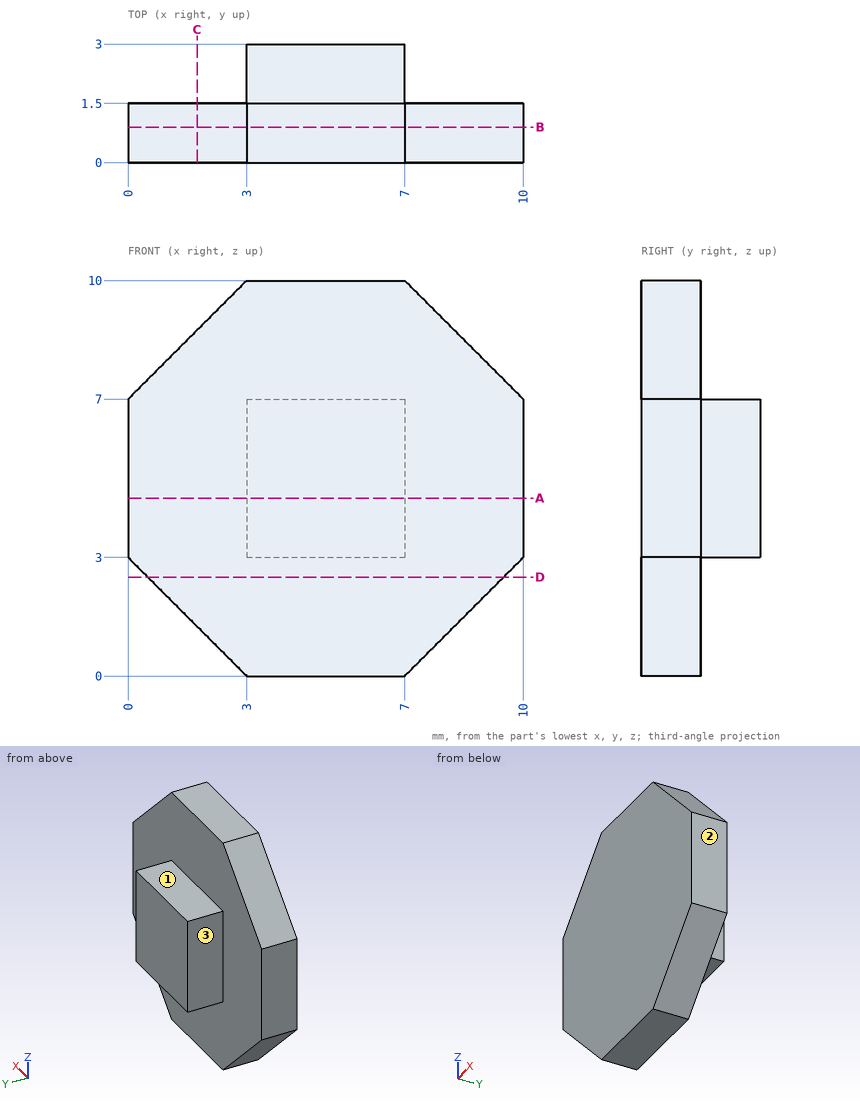
Could you check a few things on this drawing? It's one solid part, dimensions in mm from its lowest x, y, z. A direction names the side the tool comes from. Give positions to 0.01 mm unless a question says otherwise; leave off trailing zeros. Order: outer loops, then holes, each group sorted by start corner. A loop starts at its lowest first (then second) coordinate and runs counter-clockwise, first axis right, second up. Notation, with made-up numbers: M -31,54 L -6,54 A11 ccw -6,60 Z; hole C -31,-23 d7. An arc over 180 degrees is marked long. Use one line per item in the form item = value.
Item 1: If we section it at D-D, the plane z = 2.5: Write out the boundary of the cut face in (x, y), and give its area (3 significant figures).
Values follow:
outline = M 0.5,0 L 9.5,0 L 9.5,1.5 L 0.5,1.5 Z
area = 13.5 mm^2
Item 2: If I drill on line 1 along Y through (x, z) = (8.25, 1.75); line 2 along Z through (x, y) = (4.75, 2.45), over which ranges is the centre line in solid material (lowest first)? Write a range as [from, to].
Values follow:
line_1 = [0, 1.5]
line_2 = [3, 7]
Item 3: If we section it at C-C, the plane x = 1.75: Write out the boundary of the cut face in (y, z).
Values follow:
outline = M 0,1.25 L 1.5,1.25 L 1.5,8.75 L 0,8.75 Z
Item 4: Will these pins go through, and if not, where does the flat tip stop? pin 1 Ø1.5 at (x, y) = (4, 0.5) entering from -Z; pin 2 Ø0.8 at (y, z) = (2.5, 6) entering from +X; pin 3 Ø1 at (y, z) = (2.5, 8.5) entering from +X; pin 4 Ø1.2 at (y, z) = (2.5, 5) entering from -X.
Values follow:
pin_1 = 0
pin_2 = 7
pin_3 = through
pin_4 = 3
Item 5: If we section it at A-A, the plane z = 4.5: Write out the boundary of the cut face in (x, y).
Values follow:
outline = M 0,0 L 10,0 L 10,1.5 L 7,1.5 L 7,3 L 3,3 L 3,1.5 L 0,1.5 Z
Item 6: For the marked faces 1, 2 and 3, which set-ups out of +Z, -Z, +X, -X, +Y, -Y let a thin tool reach every point of the face, with its end or its side?
Values follow:
face_1 = +Z, +X, -X, +Y
face_2 = +Z, -Z, +X, +Y, -Y
face_3 = +Z, -Z, -X, +Y
Item 7: If we section it at B-B, the plane y = 0.9: Write out the boundary of the cut face in (x, z), and give its area (3 significant figures).
Values follow:
outline = M 0,3 L 3,0 L 7,0 L 10,3 L 10,7 L 7,10 L 3,10 L 0,7 Z
area = 82.0 mm^2
